Input: part model. Units: mm. Frame: model coordinates. Face numbers are marked on the shaded views. A direction names the side the tool comes from. Coordinates: 2 decimals unless noted, no trailing zeros. Loops run counter-clockwise (first coordinate to the right, second up) from the corner with the lowest first, then second, coordinate; pieces in that order, holes last.
Item 1: Section B-B on y = 135.75. Return loops of the section in (x, z), and give its area (3 significant figures).
Item 2: Section A-A on z = 1.85. Return loops of the section in (x, y).
Item 3: Section C-C on x = 211.5. Return loops of the section in (y, z) (3 decimals).
Item 4: Pull-direction query (X, two-part tool) for the marked faces 3, 4 and 5; classes: released by +X, released by -X, zero draft, split by the parting line, or undercut.
Item 5: Section D-D on x = 214. Return loops of the section in (y, z) (3 decimals), and give its area (3 significant figures).
Item 6: Reachability of the marked faces 1 and 2 from +Z, -Z, +X, -X, +Y, -Y: full face, straight path, thin tool, end or side. Return the list, or none.
Item 7: Ray query, line 1 along Y through (x, z) = (212.5, 2.4); line 2 along X through (y, z) = (135, 2.95); line 3 along Y through (x, z) = (213.25, 0.4). Return the intervals inside material, ascending.
```python
from build123d import *

# Parameters (mm, degrees)
SKETCH1_W           = 6.14482622
SKETCH1_H           = 11.373318705
BOSS_EXTRUDE1_DEPTH = 3.2
SKETCH2_R           = 1.4
CUT_EXTRUDE1_DEPTH  = 261.036225732
CUT_EXTRUDE2_DEPTH  = 145.0912201


with BuildPart() as part:
    # Sketch1 → Boss-Extrude1 (new body)
    with BuildSketch(Plane.XY):
        with Locations((213.478545955, 138.237907074)):
            Rectangle(SKETCH1_W, SKETCH1_H)
    extrude(amount=BOSS_EXTRUDE1_DEPTH)

    # Sketch2 → Cut-Extrude1 (cut, through all)
    with BuildSketch(Plane(origin=(0, 0, 0), x_dir=(-1, 0, 0), z_dir=(0, 0, -1))):
        with Locations((-213.478545955, 141.487907073)):
            Circle(SKETCH2_R)
        with Locations((-213.478545955, 134.987907073)):
            Circle(SKETCH2_R)
    extrude(amount=-CUT_EXTRUDE1_DEPTH, mode=Mode.SUBTRACT)

    # Sketch3 → Cut-Extrude2 (cut, through all)
    with BuildSketch(Plane(origin=(216.550959065, 0, 0), x_dir=(0, 0, -1), z_dir=(1, 0, 0))):
        with BuildLine():
            Line((-2.135, 137.172907073), (-3.2, 137.172907073))
            Line((-3.2, 137.172907073), (-3.2, 139.302907073))
            Line((-3.2, 139.302907073), (-2.135, 139.302907073))
            ThreePointArc((-2.135, 139.302907073), (-1.07, 138.237907073), (-2.135, 137.172907073))
        make_face()
    extrude(amount=-CUT_EXTRUDE2_DEPTH, mode=Mode.SUBTRACT)


solid = part.part
```
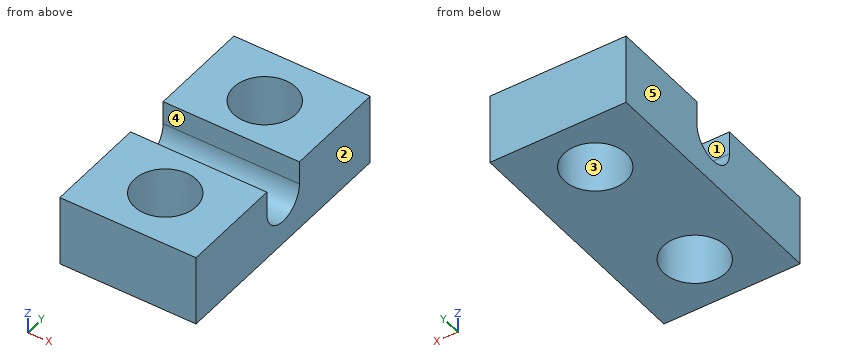
Results found:
1. outline: (210.41, 0) - (212.3, 0) - (212.3, 3.2) - (210.41, 3.2) - close; (214.65, 0) - (216.55, 0) - (216.55, 3.2) - (214.65, 3.2) - close
1. area: 12.1 mm2
2. outline: (210.41, 132.55) - (216.55, 132.55) - (216.55, 137.21) - (210.41, 137.21) - close; (210.41, 139.26) - (216.55, 139.26) - (216.55, 143.92) - (210.41, 143.92) - close; hole circle Ø2.8 at (213.48, 134.99); hole circle Ø2.8 at (213.48, 141.49)
3. outline: (132.551, 0) - (143.925, 0) - (143.925, 3.2) - (139.303, 3.2) - (139.303, 2.135) arc R1.065 cw to (137.173, 2.135) - (137.173, 3.2) - (132.551, 3.2) - close
4. face 3: undercut
4. face 4: zero draft
4. face 5: released by -X
5. outline: (132.551, 0) - (133.689, 0) - (133.689, 3.2) - (132.551, 3.2) - close; (136.287, 0) - (140.189, 0) - (140.189, 3.2) - (139.303, 3.2) - (139.303, 2.135) arc R1.065 cw to (137.173, 2.135) - (137.173, 3.2) - (136.287, 3.2) - close; (142.787, 0) - (143.925, 0) - (143.925, 3.2) - (142.787, 3.2) - close
5. area: 15.7 mm2
6. face 1: +Z, +X, -X
6. face 2: +Z, -Z, +X, +Y, -Y
7. line 1: y = 132.55 to 133.99, 135.99 to 137.17, 139.3 to 140.49, 142.49 to 143.92
7. line 2: x = 210.41 to 212.08, 214.88 to 216.55
7. line 3: y = 132.55 to 133.61, 136.37 to 140.11, 142.87 to 143.92
